Geometry check sheet. Reference: drawing and pictorial views, mm from the part's lowest x, y, z. Round coordinates to 2 decimals unless told otherwise and drop trailing zeros. Write each loop counter-clockwise with the first axis right and the second up, starting at its lowest first coordinate (ties: lowest second). Pieces come first, ordered by that corner, then holes. Notation, with made-up numbers: (0, -38.75) - (8, -38.75) arc R22 ccw to (8, -8.75) - close; hole circle Ø11 at (70, 1.25). An arc over 180 degrees is marked (long way). Return JSON: item names as keys, results as strings.
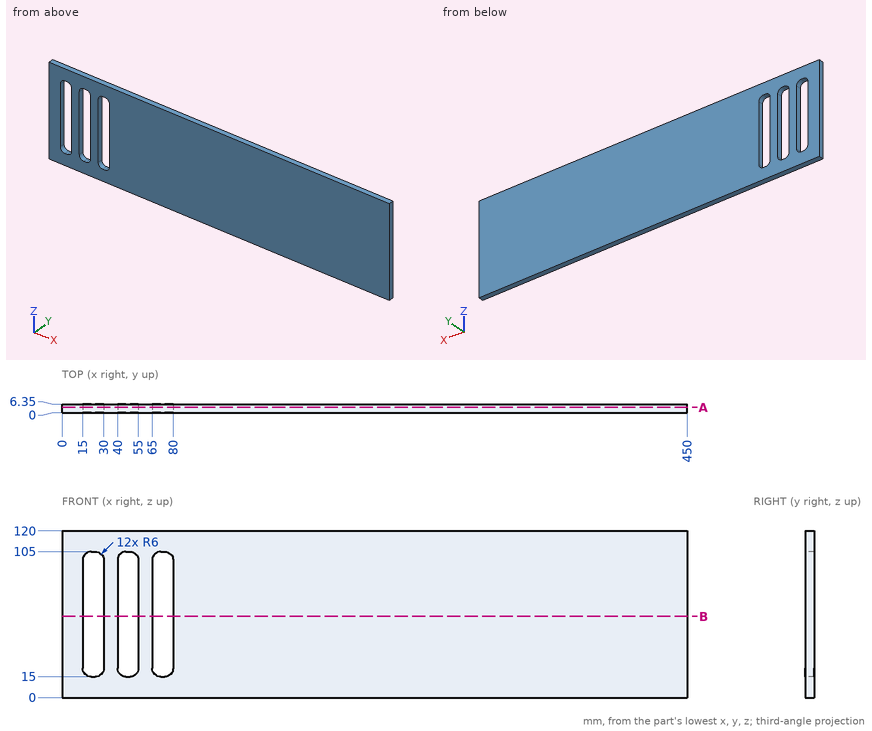
(1) Section check B-B, the plane z = 58.5. Enter the section's corners in (x, y).
Response values:
{"outline": "(0, 0) - (15, 0) - (15, 6.35) - (0, 6.35) - close; (30, 0) - (40, 0) - (40, 6.35) - (30, 6.35) - close; (55, 0) - (65, 0) - (65, 6.35) - (55, 6.35) - close; (80, 0) - (450, 0) - (450, 6.35) - (80, 6.35) - close"}
(2) Material ranges on line 1 along X through (y, z) = (5, 84); line 2 along X through (y, z) = (4.25, 16.5); line 3 along Z through (x, y) = (27, 5.5), recorded low to high. Write a range as [from, to].
Response values:
{"line 1": "x = [0, 15], [30, 40], [55, 65], [80, 450]", "line 2": "x = [0, 17.03], [27.97, 42.03], [52.97, 67.03], [77.97, 450]", "line 3": "z = [0, 15.8], [104.2, 120]"}
(3) Section check A-A, the plane y = 4. Enter the section's corners in (x, z).
Response values:
{"outline": "(0, 0) - (450, 0) - (450, 120) - (0, 120) - close; hole (15, 21) arc R6 ccw to (21, 15) - (24, 15) arc R6 ccw to (30, 21) - (30, 99) arc R6 ccw to (24, 105) - (21, 105) arc R6 ccw to (15, 99) - close; hole (40, 21) arc R6 ccw to (46, 15) - (49, 15) arc R6 ccw to (55, 21) - (55, 99) arc R6 ccw to (49, 105) - (46, 105) arc R6 ccw to (40, 99) - close; hole (65, 21) arc R6 ccw to (71, 15) - (74, 15) arc R6 ccw to (80, 21) - (80, 99) arc R6 ccw to (74, 105) - (71, 105) arc R6 ccw to (65, 99) - close"}
